from build123d import *

# Parameters (mm, degrees)
SKETCH1_W           = 10
SKETCH1_H           = 10
BOSS_EXTRUDE1_DEPTH = 10
SKETCH2_R           = 0.95
CUT_EXTRUDE1_DEPTH  = 11
SKETCH3_R           = 0.95
CUT_EXTRUDE2_DEPTH  = 11
SKETCH5_R           = 0.95
CUT_EXTRUDE4_DEPTH  = 11
CHAMFER1_SIZE       = 0.2
CHAMFER2_SIZE       = 0.1


with BuildPart() as part:
    # Sketch1 → Boss-Extrude1 (new body)
    with BuildSketch(Plane.XY):
        Rectangle(SKETCH1_W, SKETCH1_H)
    extrude(amount=BOSS_EXTRUDE1_DEPTH)

    # Sketch2 → Cut-Extrude1 (cut, through all)
    with BuildSketch(Plane.XY.offset(10)):
        with Locations((-2.5, 0)):
            Circle(SKETCH2_R)
        with Locations(Location((2.5, 0, 0), (0, 0, 180))):  # turned: the seam where the file's is
            Circle(SKETCH2_R)
    extrude(amount=-CUT_EXTRUDE1_DEPTH, mode=Mode.SUBTRACT)

    # Sketch3 → Cut-Extrude2 (cut, through all)
    with BuildSketch(Plane(origin=(0, 5, 0), x_dir=(1, 0, 0), z_dir=(0, 1, 0))):
        with Locations(Location((0, -7.5, 0), (0, 0, 90))):  # turned: the seam where the file's is
            Circle(SKETCH3_R)
        with Locations(Location((0, -2.5, 0), (0, 0, 270))):  # turned: the seam where the file's is
            Circle(SKETCH3_R)
    extrude(amount=-CUT_EXTRUDE2_DEPTH, mode=Mode.SUBTRACT)

    # Sketch5 → Cut-Extrude4 (cut, through all)
    with BuildSketch(Plane(origin=(5, 0, 0), x_dir=(0, 0, -1), z_dir=(1, 0, 0))):
        with Locations(Location((-5, 2.5, 0), (0, 0, 90))):  # turned: the seam where the file's is
            Circle(SKETCH5_R)
        with Locations(Location((-5, -2.5, 0), (0, 0, 270))):  # turned: the seam where the file's is
            Circle(SKETCH5_R)
    extrude(amount=-CUT_EXTRUDE4_DEPTH, mode=Mode.SUBTRACT)

    # Chamfer1
    chamfer1_edges = [part.edges().sort_by_distance(p)[0] for p in [
        (5, 0, 10),
        (0, 5, 10),
        (-5, 0, 10),
        (0, 5, 0),
        (5, 0, 0),
        (0, -5, 0),
        (-5, 0, 0),
        (0, -5, 10),
        (-5, 5, 5),
        (5, 5, 5),
        (5, -5, 5),
        (-5, -5, 5),
    ]]
    chamfer(chamfer1_edges, length=CHAMFER1_SIZE)

    # Chamfer2
    chamfer2_edges = [part.edges().sort_by_distance(p)[0] for p in [
        (-3.45, 0, 0),
        (-3.45, 0, 10),
        (3.45, 0, 0),
        (3.45, 0, 10),
        (0, -5, 8.45),
        (0, 5, 8.45),
        (0, -5, 1.55),
        (0, 5, 1.55),
        (-5, 1.55, 5),
        (5, 1.55, 5),
        (-5, -1.55, 5),
        (5, -1.55, 5),
    ]]
    chamfer(chamfer2_edges, length=CHAMFER2_SIZE)


solid = part.part
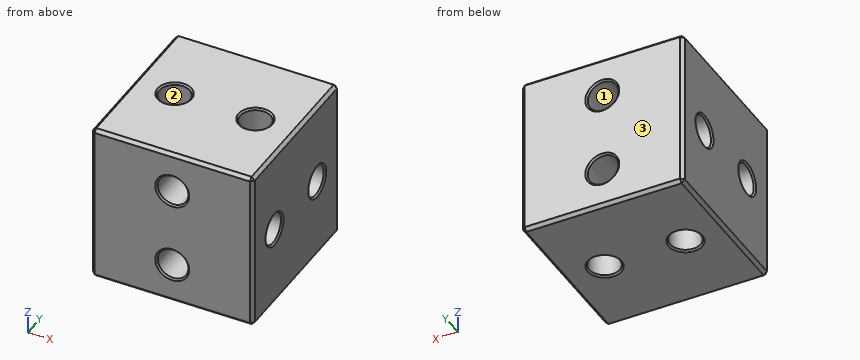
CAD build for the part. Positions are in the model's coordinates, mm. Face numbers are marked on the shaded views. Give positions to 0.01 mm unless a question says otherwise; leave off trailing zeros. Write each loop counter-clockwise with the first axis right and the second up, starting at its lowest first coordinate (ties: lowest second). Pieces come first, ordered by that corner, then holes. Notation, with made-up numbers: M -16.5,71 L 28.5,71 A22 ccw 28.5,82 Z; hole C 32.5,5.25 d8. An arc over 180 degrees is marked long. Put each result on its own line as item: value. Start each with the question number.
(1) Band-saw the part on B-B, the plane y = 0. Write the cut outline in (x, z).
(2) Band-saw the part on A-A, the plane z = 5. Write the cut outline in (x, y).
(3) Band-saw the part on D-D, the plane z = 7.5. Write the cut outline in (x, y), and give its area (3 significant figures).
(4) Mould opens along Y. For the marked faces 1, 2 and 3 say: +Y half, -Y half, draft (parallel to the pull), parting line (faces both ways), or undercut.
(5) Band-saw the part on C-C, the plane x = -2.5. Write the cut outline in (y, z).
(6) Probe L1, parallel to Z at x = -3.75, y = -2.5; L2, parallel to X at y = -0.25, z = 2.5; L3, parallel to X at y = 1.5, z = 7.5. List the from-to ranges inside material, lowest first.
Response values:
1. outline: M -5,0.2 L -4.8,0 L -3.55,0 L -3.45,0.1 L -3.45,9.9 L -3.55,10 L -4.8,10 L -5,9.8 Z; M -1.55,0.1 L -1.45,0 L 1.45,0 L 1.55,0.1 L 1.55,9.9 L 1.45,10 L -1.45,10 L -1.55,9.9 Z; M 3.45,0.1 L 3.55,0 L 4.8,0 L 5,0.2 L 5,9.8 L 4.8,10 L 3.55,10 L 3.45,9.9 Z; hole C 0,2.5 d1.9; hole C 0,7.5 d1.9
2. outline: M -5,-4.8 L -4.8,-5 L 4.8,-5 L 5,-4.8 L 5,-3.55 L 4.9,-3.45 L -4.9,-3.45 L -5,-3.55 Z; M -5,-1.45 L -4.9,-1.55 L 4.9,-1.55 L 5,-1.45 L 5,1.45 L 4.9,1.55 L -4.9,1.55 L -5,1.45 Z; M -5,3.55 L -4.9,3.45 L 4.9,3.45 L 5,3.55 L 5,4.8 L 4.8,5 L -4.8,5 L -5,4.8 Z; hole C -2.5,0 d1.9; hole C 2.5,0 d1.9
3. outline: M -5,-4.8 L -4.8,-5 L -1.05,-5 L -0.95,-4.9 L -0.95,4.9 L -1.05,5 L -4.8,5 L -5,4.8 Z; M 0.95,-4.9 L 1.05,-5 L 4.8,-5 L 5,-4.8 L 5,4.8 L 4.8,5 L 1.05,5 L 0.95,4.9 Z; hole C -2.5,0 d1.9; hole C 2.5,0 d1.9
3. area: 75.2 mm2
4. face 1: draft
4. face 2: undercut
4. face 3: +Y half
5. outline: M -5,0.2 L -4.8,0 L -1.05,0 L -0.95,0.1 L -0.95,9.9 L -1.05,10 L -4.8,10 L -5,9.8 Z; M 0.95,0.1 L 1.05,0 L 4.8,0 L 5,0.2 L 5,9.8 L 4.8,10 L 1.05,10 L 0.95,9.9 Z; hole C -2.5,5 d1.9; hole C 2.5,5 d1.9
6. L1: z = 0 to 4.05, 5.95 to 10
6. L2: x = -5 to -3.42, -1.58 to -0.95, 0.95 to 1.58, 3.42 to 5
6. L3: x = -5 to -0.95, 0.95 to 5
